```python
from build123d import *

# Parameters (mm, degrees)
BOSS_EXTRU_1_DEPTH = 2
CONG_1_R           = 4
CONG_2_R           = 1


with BuildPart() as part:
    # Esquisse1 → Boss.-Extru.1 (new body)
    with BuildSketch(Plane.XY):
        Polygon((0, 6.25), (3.541451884, 6.25), (3.541451884, 5.25), (8.641451884, 5.25), (8.641451884, 5.45), (12.082903769, 5.25), (12.082903769, -5.25), (8.641451884, -5.45), (8.641451884, -5.25), (3.541451884, -5.25), (3.541451884, -6.25), (0, -6.25), align=None)
        Polygon((2, 0), (4.020725942, -3.5), (8.062177826, -3.5), (10.082903769, 0), (8.062177826, 3.5), (4.020725942, 3.5), align=None, mode=Mode.SUBTRACT)
    extrude(amount=BOSS_EXTRU_1_DEPTH)

    # Congé1
    # the kernel refuses this fillet: 4 mm, written as the material it takes off along each edge
    with BuildSketch(Plane(origin=(0, -6.25, -9.934074449), x_dir=(1, 0, 0), z_dir=(0, 0, 1))) as cong_1_piece_1:
        with BuildLine():
            CenterArc((4, 3.97362978), CONG_1_R, 180, 83.417310117)
            Line((0, 3.97362978), (-0.08, 3.97362978))
            Line((-0.08, 3.97362978), (-0.08, 0))
            Line((-0.08, 0), (0, -0.08))
            ThreePointArc((0, -0.08), (1.770725942, -0.08), (3.532280922, -0.079472596))
            Line((3.532280922, -0.079472596), (3.541451884, 0))
        make_face()
    extrude(amount=21.868148898, mode=Mode.SUBTRACT)
    with BuildSketch(Plane(origin=(0, 6.25, -9.934074449), x_dir=(1, 0, 0), z_dir=(0, 0, 1))) as cong_1_piece_2:
        with BuildLine():
            CenterArc((4, -3.97362978), CONG_1_R, 96.582689883, 83.417310117)
            Line((0, -3.97362978), (-0.08, -3.97362978))
            Line((-0.08, -3.97362978), (-0.08, 0))
            Line((-0.08, 0), (0, 0.08))
            ThreePointArc((0, 0.08), (1.770725942, 0.08), (3.532280922, 0.079472596))
            Line((3.532280922, 0.079472596), (3.541451884, 0))
        make_face()
    extrude(amount=21.868148898, mode=Mode.SUBTRACT)

    # Congé2
    cong_2_edges = [part.edges().sort_by_distance(p)[0] for p in [
        (12.082903769, 5.25, 1),
        (12.082903769, -5.25, 1),
    ]]
    fillet(cong_2_edges, radius=CONG_2_R)


solid = part.part
```
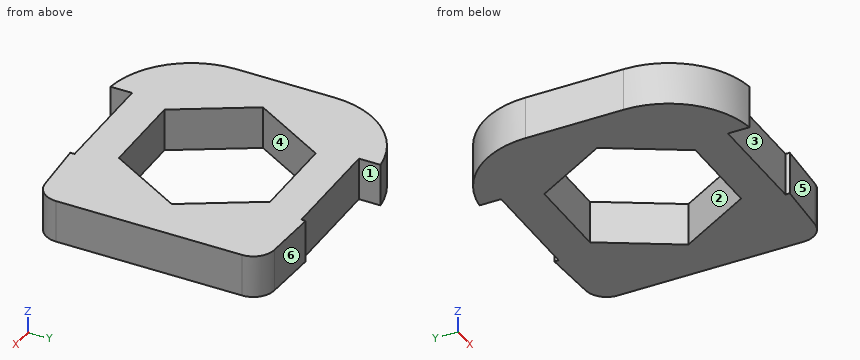
Input: part model. Units: mm. Frame: model coordinates. Face numbers are marked on the shaded views. A direction names the side the tool comes from. Give positions to 0.01 mm unless a question says otherwise; leave off trailing zeros. Order: outer loops, then holes, each group sorted by start corner. A loop starts at its lowest first (then second) coordinate and runs counter-clockwise, first axis right, second up. Notation, with made-up numbers: (-38, 31.25) - (-15, 31.25) arc R13 ccw to (-15, 54.25) - close; hole circle Ø7 at (20.5, 30.25). An arc over 180 degrees is marked (long way). Put each result on its own line as item: value.
Item 1: Draft query along Y for the marked faces 4, 5 and 6. Return one class per face: +Y half, -Y half, draft (parallel to the pull), parting line (faces both ways), or undercut.
Found:
face 4: undercut
face 5: -Y half
face 6: +Y half
Item 2: Section query B-B, the plane y = -2.75. Return loops of the section in (x, z).
Found:
outline: (0.03, 0) - (3.59, 0) - (3.59, 2) - (0.03, 2) - close; (8.5, 0) - (12.08, 0) - (12.08, 2) - (8.5, 2) - close
Item 3: Section query A-A, the plane x = 3. Return loops of the section in (y, z).
Found:
outline: (-6.15, 0) - (-1.73, 0) - (-1.73, 2) - (-6.15, 2) - close; (1.73, 0) - (6.15, 0) - (6.15, 2) - (1.73, 2) - close
Item 4: Access query for the marked faces 1, 2 and 3. Directions: +Z, -Z, +X, -X, +Y, -Y. A direction counts if a zero-diameter tool reaches every point of the face in a straight line with its end or side. Return the directions, or none.
Found:
face 1: +Z, -Z, +Y
face 2: +Z, -Z
face 3: +Z, -Z, -Y
Item 5: Section query D-D, the plane y = 5. Return loops of the section in (x, z).
Found:
outline: (1.07, 0) - (11.8, 0) - (11.8, 2) - (1.07, 2) - close
Item 6: Contact query for flat-ended pins moving along their axis: pin 1 (0.8 mm diameter, centred on y = 6, z = 1.5, fed in from +X); pin 2 (0.6 mm diameter, centred on x = 6.5, z = 0.5, fed in from -Y); pin 3 (0.6 mm diameter, centred on x = 6, z = 0.5, fed in from +Y). Output: stop coordinate, or through.
Found:
pin 1: stops at x = 3.54
pin 2: stops at y = -5.25
pin 3: stops at y = 5.25
Item 7: Ray query, L1, parallel to Y at x = 5.75, z = 0.7; L2, parallel to X at y = -3.25, z = 0.5; L3, parallel to X at y = 1.25, z = 0.8. Return the intervals inside material, ascending. Write a range as from..to.
Found:
L1: y = -5.25..-3.5, 3.5..5.25
L2: x = 0.12..3.88, 8.21..12.08
L3: x = 0..2.72, 9.36..12.08
Item 8: Section query C-C, the plane z = 1.3. Return loops of the section in (x, y), then the cut area to 3 significant figures.
Found:
outline: (0, -2.28) arc R4 ccw to (3.54, -6.25) - (3.54, -5.25) - (8.64, -5.25) - (8.64, -5.45) - (11.14, -5.3) arc R1 ccw to (12.08, -4.31) - (12.08, 4.31) arc R1 ccw to (11.14, 5.3) - (8.64, 5.45) - (8.64, 5.25) - (3.54, 5.25) - (3.54, 6.25) arc R4 ccw to (0, 2.28) - close; hole (2, 0) - (4.02, -3.5) - (8.06, -3.5) - (10.08, 0) - (8.06, 3.5) - (4.02, 3.5) - close
area: 85.2 mm^2
